Verification items for this drawing (mm, ordinates from the low corner). Coordinates: 2 decimals unless noted, no trailing zeros. Write each loop counter-clockwise with the first axis right and the second up, starting at its lowest first coordinate (ties: lowest second). Pieces come first, ordered by that corner, then holes. Notation, with made-up numbers: (-4, -0.5) -> (25, -0.5) arc R19 ccw to (25, 18.5) -> close; hole circle Ø6 at (13.5, 34). An arc over 180 degrees is marked (long way). One line per item, written item: value. Start each with the question number.
1) Draft check along Z on the marked faces 1, 2, 3 and 4. Enter one of: +Z half, -Z half, draft (parallel to the pull), parting line (faces both ways), or undercut.
2) Scan lines: line 1 along Z through (x, y) = (28, 0.3); line 2 along Y through (x, z) = (6.5, 26.5). Record each from-to range of solid material in increasing order. Write a range as [from, to].
3) Sectioned sample at A-A on z = 10.5. Enter the section's corners in (x, y), plus the area to 3 significant figures.
4) Sectioned sample at B-B on x = 6. Enter the section's corners in (y, z), plus the area to 3 significant figures.
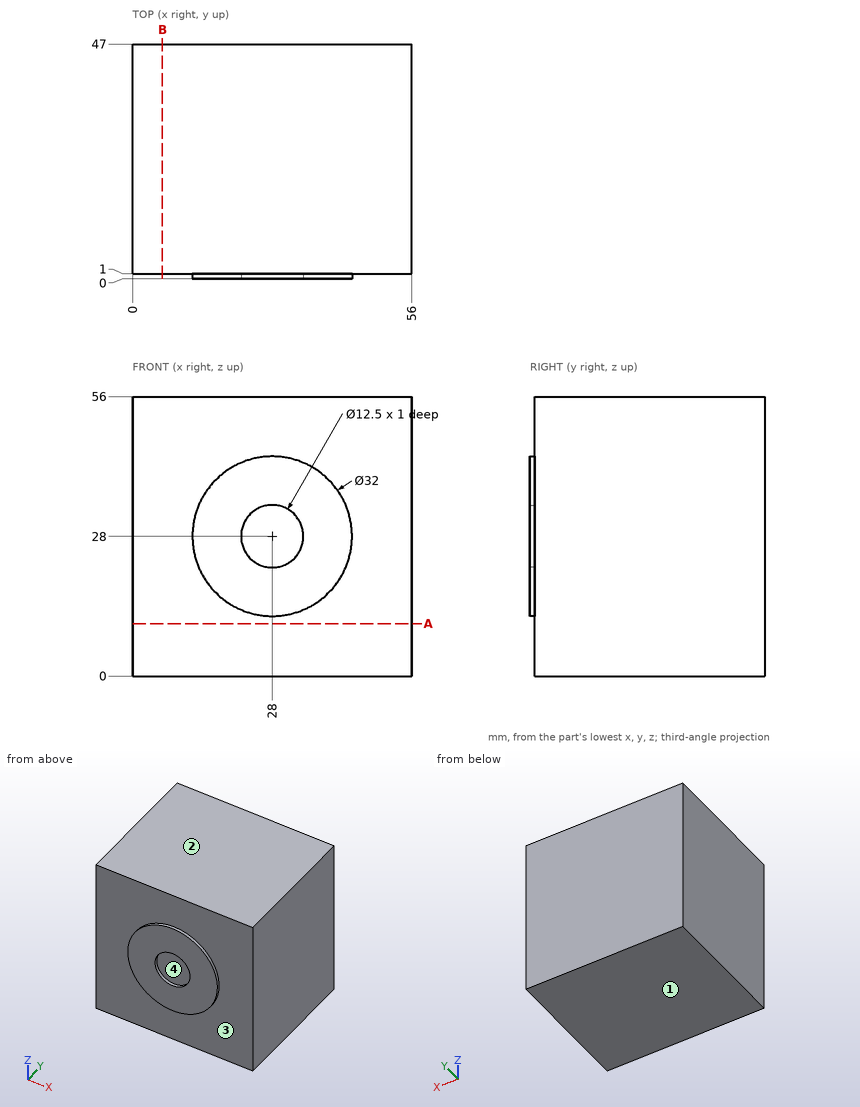
Answers:
1. face 1: -Z half
1. face 2: +Z half
1. face 3: draft
1. face 4: undercut
2. line 1: z = [12, 21.75], [34.25, 44]
2. line 2: y = [1, 47]
3. outline: (0, 1) -> (56, 1) -> (56, 47) -> (0, 47) -> close
3. area: 2,580 mm2
4. outline: (1, 0) -> (47, 0) -> (47, 56) -> (1, 56) -> close
4. area: 2,580 mm2
